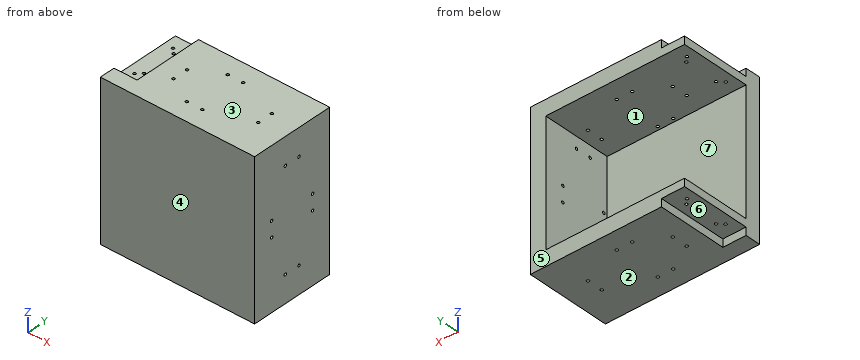
Autodesk Inventor part; units mm, degrees
ref_plane "YZ Plane" through (0, 0, 0) normal (1, 0, 0) x (0, 1, 0)
ref_plane "XZ Plane" through (0, 0, 0) normal (0, 1, 0) x (-1, 0, 0)
ref_plane "XY Plane" through (0, 0, 0) normal (0, 0, 1) x (1, 0, 0)
sketch "Boceto2" plane through (0, 0, 0) normal (0, 1, 0) x (-1, 0, 0)
  line L0 (7.5, 100) -> (-7.5, 100)
  line L1 (-7.5, 100) -> (-7.5, -100)
  line L2 (-7.5, -100) -> (7.5, -100)
  line L3 (7.5, -100) -> (7.5, 100)
  line L4 (7.5, 100) -> (-7.5, -100) construction
  line L5 (-7.5, 100) -> (7.5, -100) construction
  point P0 (0, 0)
  dimension "d7" = 15
  dimension "d8" = 200
extrude "Extrusión1" add sketch "Boceto2" along normal blind 10
sketch "Boceto3" plane through (0, 10, 0) normal (0, 1, 0) x (1, 0, 0)
  line L0 (5, 60) -> (-5, 60)
  line L1 (-5, 60) -> (-5, 70)
  line L2 (-5, 70) -> (5, 70)
  line L3 (5, 70) -> (5, 60)
  line L4 (5, 60) -> (-5, 70) construction
  line L5 (7.5, 100) -> (-7.5, 100)
  line L6 (0, 64.5148) -> (0, 61.9205)
  circle A0 centre (3.25, 61.75) radius 1.75
  circle A1 centre (-3.25, 68.25) radius 1.75
  line L7 (-7.5, 100) -> (-7.5, -100)
  line L8 (-7.5, 0) -> (0, 0)
  line L9 (5, -70) -> (5, -60)
  line L10 (-5, -70) -> (5, -70)
  line L11 (5, -60) -> (-5, -60)
  line L12 (-5, -60) -> (-5, -70)
  line L13 (5, -60) -> (-5, -70) construction
  line L14 (0, -64.5148) -> (0, -61.9205)
  circle A2 centre (-3.25, -68.25) radius 1.75
  circle A3 centre (3.25, -61.75) radius 1.75
  point P0 (3.25, 68.25)
  point P1 (-5, 65)
  point P2 (-3.25, 61.75)
  point P3 (0, 100)
  point P4 (3.25, -68.25)
  point P5 (-3.25, -61.75)
  point P6 (-5, -65)
  dimension "d12" = 1.75
  dimension "d13" = 1.75
  dimension "d14" = 1.75
  dimension "d15" = 1.75
  dimension "d16" = 10
  dimension "d17" = 10
  dimension "d19" = 30
  dimension "d67" = 31.75
hole "Agujero1" at (3.25, 10, -61.75) at (-3.25, 10, -68.25) at (-3.25, 10, 68.25) at (3.25, 10, 61.75) direction (0, -1, 0) diameter 3.5 end through all
sketch "Boceto4" plane through (0, 10, 0) normal (0, 1, 0) x (1, 0, 0)
  line L0 (-7.5, 100) -> (-7.5, -100)
  line L1 (-7.5, -100) -> (7.5, -100)
  line L2 (7.5, -100) -> (7.5, -80)
  line L3 (7.5, -80) -> (-7.5, -80)
  line L4 (-7.5, -80) -> (-7.5, -100)
  line L5 (-7.5, 0) -> (1.0116, 0)
  line L6 (-7.5, -100) -> (-7.5, 100)
  line L7 (-7.5, 100) -> (7.5, 100)
  line L8 (7.5, 100) -> (7.5, 80)
  line L9 (7.5, 80) -> (-7.5, 80)
  line L10 (-7.5, 80) -> (-7.5, 100)
  point P0 (0, 0)
  point P1 (-7.5, -80)
  point P2 (-7.5, 80)
  dimension "d27" = 15
  dimension "d28" = 20
extrude "Extrusión2" add sketch "Boceto4" along normal blind 80
sketch "Boceto5" plane through (0, 90, 0) normal (0, 1, 0) x (1, 0, 0)
  line L0 (-7.5, -100) -> (7.5, -100)
  line L1 (-7.5, -100) -> (40.5, -100)
  line L2 (40.5, -100) -> (40.5, 100)
  line L3 (40.5, 100) -> (-7.5, 100)
  line L4 (-7.5, 100) -> (-7.5, -100)
  line L5 (40.5, -100) -> (-159.5, -100)
  line L6 (-159.5, -100) -> (-159.5, 100)
  line L7 (-159.5, 100) -> (40.5, 100)
  line L8 (40.5, 100) -> (40.5, -100)
  point P0 (0, 0)
  point P1 (-7.5, 100)
  dimension "d31" = 48
  dimension "d32" = 200
  dimension "d74" = 200
extrude "Extrusión3" add sketch "Boceto5" along normal blind 110
sketch "Boceto6" plane through (0, 200, 0) normal (0, 1, 0) x (1, 0, 0)
  line L0 (40.5, 100) -> (7.5, 100)
  line L1 (40.5, 100) -> (20.5, 100)
  line L2 (20.5, 100) -> (20.5, 80)
  line L3 (7.5, -100) -> (40.5, -100)
  line L4 (24, -100) -> (24, -80)
  line L5 (-159.5, 100) -> (-159.5, -100)
  line L6 (20.5, 80) -> (-159.5, 80)
  line L7 (-159.5, 80) -> (-159.5, -80)
  line L8 (-159.5, -80) -> (20.5, -80)
  line L9 (20.5, -80) -> (20.5, 80)
  line L10 (-159.5, -100) -> (40.5, -100)
  point P0 (7.5, 80)
  point P1 (-159.5, 80)
  dimension "d36" = 20
  dimension "d37" = 20
  dimension "d38" = 20
  dimension "d78" = 20
extrude "Extrusión4" cut sketch "Boceto6" against normal blind 90
sketch "Boceto7" plane through (-159.5, 90, -100) normal (-1, 0, 0) x (0, 0, 1)
  line L0 (0, 110) -> (20, 110)
  line L1 (20, 110) -> (10, 110)
  line L2 (10, 110) -> (10, 20)
  line L3 (10, 20) -> (20, 20)
  line L4 (20, 20) -> (20, 110)
  line L5 (180, 110) -> (180, 20)
  line L6 (180, 110) -> (190, 110)
  line L7 (190, 110) -> (190, 20)
  line L8 (190, 20) -> (180, 20)
  line L9 (180, 20) -> (180, 110)
  line L10 (200, 0) -> (200, 110)
  line L11 (0, 0) -> (0, 110)
  line L12 (0, 110) -> (10, 110)
  line L13 (10, 110) -> (10, 20)
  line L14 (10, 20) -> (0, 20)
  line L15 (0, 20) -> (0, 110)
  line L16 (200, 110) -> (0, 110)
  line L17 (200, 110) -> (190, 110)
  line L18 (190, 110) -> (190, 20)
  line L19 (190, 20) -> (200, 20)
  line L20 (200, 20) -> (200, 110)
  point P0 (100, -90)
  point P1 (200, 20)
  dimension "d42" = 10
  dimension "d63" = 10
  dimension "d65" = 10
extrude "Extrusión5" cut sketch "Boceto7" against normal blind 30 contours L0 L2 L14 L11 | L16 L10 L19 L7
sketch "Boceto8" plane through (-7.5, 0, 100) normal (0, 0, 1) x (1, 0, 0)
  line L0 (-122, 200) -> (-122, 110)
  line L1 (-132, 175) -> (-142, 175)
  line L2 (-142, 175) -> (-142, 185)
  line L3 (-142, 185) -> (-132, 185)
  line L4 (-132, 185) -> (-132, 175)
  line L5 (-132, 175) -> (-142, 185) construction
  line L6 (-142, 175) -> (-132, 185) construction
  line L7 (-152, 200) -> (48, 200)
  line L8 (-113, 155) -> (-128, 155)
  line L9 (-152, 110) -> (-122, 110)
  line L10 (-132, 180) -> (-131.5898, 180)
  circle A0 centre (-140.25, 183.25) radius 1.75
  circle A1 centre (-133.75, 176.75) radius 1.75
  line L11 (-132, 125) -> (-132, 135)
  line L12 (-142, 125) -> (-132, 125)
  line L13 (-132, 135) -> (-142, 125) construction
  line L14 (-132, 135) -> (-142, 135)
  line L15 (-142, 135) -> (-132, 125) construction
  line L16 (-142, 135) -> (-142, 125)
  line L17 (-132, 130) -> (-131.5898, 130)
  circle A2 centre (-133.75, 133.25) radius 1.75
  circle A3 centre (-140.25, 126.75) radius 1.75
  line L18 (-152, 110) -> (-152, 200)
  point P0 (7.5, 0)
  point P1 (-113, 215)
  point P2 (-133.75, 183.25)
  point P3 (-142, 180)
  point P4 (-140.25, 176.75)
  point P5 (48, 200)
  point P6 (-133.75, 126.75)
  point P7 (-140.25, 133.25)
  point P8 (-143, 115)
  point P9 (-133.75, 126.75)
  point P10 (-140.25, 133.25)
  point P11 (-142, 130)
  dimension "d46" = 1.75
  dimension "d47" = 1.75
  dimension "d48" = 1.75
  dimension "d49" = 1.75
  dimension "d50" = 10
  dimension "d51" = 10
  dimension "d52" = 15
  dimension "d66" = 10
  dimension "d70" = 15
hole "Agujero2" at (-147.75, 183.25, 100) at (-141.25, 176.75, 100) at (-147.75, 126.75, 100) at (-141.25, 133.25, 100) direction (0, 0, -1) diameter 3.5 end through all
ref_plane "Plano de trabajo1" through (-159.5, 90, 100) normal (0, -1, 0) x (1, 0, 0)
split "Dividir1" plane through (-159.5, 90, 100) removes the side toward (0, -1, 0)
ref_plane "Plano de trabajo2" through (-159.5, 200, 0) normal (0, 0, 1) x (1, 0, 0)
ref_plane "Plano de trabajo3" through (-59.5, 90, 100) normal (1, 0, 0) x (0, 0, -1)
sketch "Boceto9" plane through (-159.5, 90, 100) normal (0, 0, 1) x (1, 0, 0)
  line L0 (85.0357, 30) -> (115.0357, 30)
  circle A0 centre (110.0357, 25) radius 1.75
  line L1 (90.0357, 25) -> (110.0357, 25)
  line L2 (115.0357, 30) -> (115.0357, 20)
  circle A1 centre (90.0357, 25) radius 1.75
  line L3 (85.0357, 20) -> (115.0357, 30) construction
  line L4 (85.0357, 30) -> (115.0357, 20) construction
  line L5 (85.0357, 20) -> (85.0357, 30)
  line L6 (115.0357, 20) -> (85.0357, 20)
  line L7 (240, 0) -> (-40, 0)
  line L8 (200, 0) -> (200, 110)
  line L9 (200, 55) -> (88.2857, 55)
  line L10 (85.0357, 80) -> (115.0357, 80)
  circle A2 centre (110.0357, 85) radius 1.75
  line L11 (90.0357, 85) -> (110.0357, 85)
  line L12 (115.0357, 80) -> (115.0357, 90)
  circle A3 centre (90.0357, 85) radius 1.75
  line L13 (85.0357, 90) -> (115.0357, 80) construction
  line L14 (85.0357, 80) -> (115.0357, 90) construction
  line L15 (85.0357, 90) -> (85.0357, 80)
  line L16 (115.0357, 90) -> (85.0357, 90)
  line L17 (100.0357, 55) -> (185.099, 55) construction
  line L18 (160, 70) -> (160, 40)
  circle A4 centre (165, 45) radius 1.75
  line L19 (165, 65) -> (165, 45)
  line L20 (160, 40) -> (170, 40)
  circle A5 centre (165, 65) radius 1.75
  line L21 (170, 70) -> (160, 40) construction
  line L22 (160, 70) -> (170, 40) construction
  line L23 (170, 70) -> (160, 70)
  line L24 (170, 40) -> (170, 70)
  circle A6 centre (55, 65) radius 1.75
  line L25 (60, 70) -> (60, 40)
  line L26 (60, 70) -> (50, 40) construction
  line L27 (50, 70) -> (60, 70)
  line L28 (50, 40) -> (50, 70)
  line L29 (50, 70) -> (60, 40) construction
  circle A7 centre (55, 45) radius 1.75
  line L30 (55, 65) -> (55, 45)
  line L31 (60, 40) -> (50, 40)
  line L32 (30, 110) -> (30, 20)
  point P0 (159.5, -90)
  point P1 (100.0357, 34.7141)
  point P2 (85.0357, 36.6749)
  point P3 (100.0357, 34.7141)
  point P4 (115.0357, 25)
  point P5 (115.0357, 85)
  point P6 (189.1833, 40)
  point P7 (165, 70)
  point P8 (70.0357, 40)
  point P9 (55, 70)
  dimension "d83" = 10
  dimension "d84" = 30
  dimension "d85" = 5
  dimension "d86" = 5
  dimension "d87" = 5
  dimension "d88" = 5
  dimension "d89" = 20
  dimension "d91" = 30
  dimension "d92" = 5
  dimension "d93" = 5
  dimension "d94" = 3.5
  dimension "d95" = 5
  dimension "d96" = 5
  dimension "d97" = 5
  dimension "d98" = 5
  dimension "d99" = 5
  dimension "d100" = 20
ref_plane "Plano de trabajo4" through (0, 145, 0) normal (0, 1, 0) x (1, 0, 0)
hole "Agujero3" at (-104.5, 155, 100) at (-69.4643, 175, 100) at (-49.4643, 175, 100) at (-104.5, 135, 100) at (-69.4643, 115, 100) at (-49.4643, 115, 100) at (5.5, 135, 100) at (5.5, 155, 100) direction (0, 0, -1) diameter 3.5 end through all
sketch "Boceto10" plane through (40.5, 90, 100) normal (1, 0, 0) x (0, 0, -1)
  line L0 (85.0357, 30) -> (115.0357, 30)
  circle A0 centre (110.0357, 25) radius 1.75
  line L1 (90.0357, 25) -> (110.0357, 25)
  line L2 (115.0357, 30) -> (115.0357, 20)
  circle A1 centre (90.0357, 25) radius 1.75
  line L3 (85.0357, 20) -> (115.0357, 30) construction
  line L4 (85.0357, 30) -> (115.0357, 20) construction
  line L5 (85.0357, 20) -> (85.0357, 30)
  line L6 (115.0357, 20) -> (85.0357, 20)
  circle A2 centre (90.0357, 85) radius 1.75
  line L7 (85.0357, 80) -> (115.0357, 80)
  line L8 (85.0357, 80) -> (115.0357, 90) construction
  line L9 (85.0357, 90) -> (85.0357, 80)
  line L10 (115.0357, 90) -> (85.0357, 90)
  line L11 (85.0357, 90) -> (115.0357, 80) construction
  circle A3 centre (110.0357, 85) radius 1.75
  line L12 (90.0357, 85) -> (110.0357, 85)
  line L13 (115.0357, 80) -> (115.0357, 90)
  line L14 (160, 70) -> (160, 40)
  circle A4 centre (165, 45) radius 1.75
  line L15 (170, 40) -> (170, 70)
  line L16 (170, 70) -> (160, 40) construction
  line L17 (160, 40) -> (170, 40)
  line L18 (160, 70) -> (170, 40) construction
  circle A5 centre (165, 65) radius 1.75
  line L19 (165, 65) -> (165, 45)
  line L20 (170, 70) -> (160, 70)
  circle A6 centre (35, 65) radius 1.75
  line L21 (40, 70) -> (40, 40)
  line L22 (40, 40) -> (30, 40)
  circle A7 centre (35, 45) radius 1.75
  line L23 (35, 65) -> (35, 45)
  line L24 (40, 70) -> (30, 40) construction
  line L25 (30, 40) -> (30, 70)
  line L26 (30, 70) -> (40, 40) construction
  line L27 (30, 70) -> (40, 70)
  line L28 (0, 0) -> (0, 110)
  line L29 (200, 0) -> (200, 110)
  point P0 (100, -90)
  point P1 (100.0357, 34.7141)
  point P2 (100.0357, 34.7141)
  point P3 (85.0357, 36.6749)
  point P4 (115.0357, 25)
  point P5 (88.2857, 55)
  point P6 (115.0357, 85)
  point P7 (100.0357, 55)
  point P8 (189.1833, 40)
  point P9 (165, 70)
  point P10 (70.0357, 40)
  point P11 (35, 70)
  dimension "d108" = 10
  dimension "d109" = 30
  dimension "d110" = 5
  dimension "d111" = 5
  dimension "d112" = 5
  dimension "d113" = 5
  dimension "d114" = 5
  dimension "d115" = 5
  dimension "d116" = 3.5
  dimension "d117" = 5
  dimension "d118" = 5
  dimension "d119" = 5
  dimension "d120" = 5
  dimension "d121" = 5
  dimension "d122" = 30
  dimension "d123" = 30
hole "Agujero4" at (40.5, 175, 9.9643) at (40.5, 175, -10.0357) at (40.5, 155, 65) at (40.5, 135, 65) at (40.5, 115, 9.9643) at (40.5, 115, -10.0357) at (40.5, 135, -65) at (40.5, 155, -65) direction (-1, 0, 0) diameter 3.5 end through all
properties part number "container_back_head"
Verification items for the finished model (mm, model axes). Face numbers are marked on the shaded views. A direction names the side the tool comes from. Coordinates: 2 decimals unless noted, no trailing zeros. Loops run counter-clockwise (first coordinate to the right, second up) from the corner with the lowest first, then second, coordinate; pieces in that order, holes last. Notation, with made-up numbers: (16, 67.5) -> (51, 67.5) arc R21 ccw to (51, 99.5) -> close; hole circle Ø8 at (69, -11.75). An arc over 180 degrees is marked (long way). Put each result on its own line as item: value.
1. Thickness scan on line 1 (Y direction, x = 30, z = 65); line 2 (X direction, y = 115, z = 87.5); line 3 (Z direction, x = 26, y = 175). Record the ranges inside material, lowest first.
Result set:
line 1: y = 90 to 133.25, 136.75 to 153.25, 156.75 to 200
line 2: x = -159.5 to -71.21, -67.71 to -51.21, -47.71 to 40.5
line 3: z = -100 to -11.79, -8.29 to 8.21, 11.71 to 100
2. Mould release check, pull along Z, two halves, no side actions. Record for the marked faces 1, 2, 3 and 4: pulls with the +Z half, pulls with the -Z half, needs draft (parallel to the pull), parting line crosses it, or undercut.
Result set:
face 1: undercut
face 2: pulls with the -Z half
face 3: pulls with the +Z half
face 4: needs draft
3. Section check C-C, the plane z = 16. Record the boundary of the cut face in (x, y), then the cut area to 3 significant figures.
Result set:
outline: (-159.5, 90) -> (40.5, 90) -> (40.5, 200) -> (20.5, 200) -> (20.5, 110) -> (-159.5, 110) -> close
area: 5,800 mm^2
4. Section check B-B, the plane y = 121.5. Record the boundary of the cut face in (x, z), then the cut area to 3 significant figures.
Result set:
outline: (-159.5, -90) -> (-129.5, -90) -> (-129.5, -100) -> (40.5, -100) -> (40.5, 100) -> (-129.5, 100) -> (-129.5, 90) -> (-159.5, 90) -> (-159.5, 80) -> (20.5, 80) -> (20.5, -80) -> (-159.5, -80) -> close
area: 10,600 mm^2
5. Gauge pin test, flat ends, axial feed: P1, Ø10, axis at y = 166.5, z = 43, coming from the -X side; P2, Ø3, axis at y = 135, z = -65, coming from the -X side; P3, Ø4, axis at x = -141.25, y = 133.25, coming from the +Z side. Record the tip position at first contact, or that the pin passes through.
Result set:
P1: stops at x = 20.5
P2: passes through
P3: stops at z = 90
6. Section check A-A, the plane x = -62. Record the boundary of the cut face in (y, z).
Result set:
outline: (90, -100) -> (200, -100) -> (200, -80) -> (110, -80) -> (110, 80) -> (200, 80) -> (200, 100) -> (90, 100) -> close
7. Tool access check on the marked faces 5, 6 and 7. Record the directions out of +Z, -Z, +X, -X, +Y, -Y that give a thin tool (end or side, any length) a straight path to the whole face; none if there is none.
Result set:
face 5: +Z, -Z, +X, -X, +Y
face 6: -Z, -X, +Y
face 7: -X, +Y
